Work out the finished part from the listing and answer in its coordinate system (mm). A direction names the side the tool comes from. Give positions to 0.01 mm unless a question says otherwise; leave off trailing zeros. Loops run counter-clockwise (first coordinate to the right, second up) from the corner with the lowest first, then second, coordinate; pieces in that order, holes last. Notation, with made-up numbers: (-25.5, -26) - (-11.5, -26) arc R24 cw to (-11.5, 10) - close; hole circle Ø5 at (52.25, 71.25). An arc over 180 degrees is marked (long way). Use CSV: the item, a comma, the result in double quotes.
from build123d import *

# Parameters (mm, degrees)
BOSS_EXTRU_1_DEPTH = 6.9
TROU_TARAUD_M81_D  = 6.8


with BuildPart() as part:
    # Esquisse1 → Boss.-Extru.1 (new body)
    with BuildSketch(Plane.XY):
        Polygon((-5.9, -3.406366588), (0, -6.812733176), (5.9, -3.406366588), (5.9, 3.406366588), (0, 6.812733176), (-5.9, 3.406366588), align=None)
    extrude(amount=BOSS_EXTRU_1_DEPTH)

    # Esquisse2 → Révolution1 (revolve)
    with BuildSketch(Plane(origin=(0, 0, 0), x_dir=(0, 0, -1), z_dir=(1, 0, 0)), mode=Mode.PRIVATE) as r_volution1_sk:
        Polygon((-1, 8.4), (-2.5, 5.801923789), (-2.5, 0), (0, 0), (0, 8.4), align=None)
    revolve(r_volution1_sk.sketch.rotate(Axis((0, 0, 0), (0, 0, 1)), 90), axis=Axis((0, 0, 0), (0, 0, 1)))

    # Esquisse3 → Enlèvement de matière-Révolution1 (revolve, cut)
    with BuildSketch(Plane(origin=(0, 0, 0), x_dir=(0, 0, -1), z_dir=(1, 0, 0))):
        Polygon((-6.9, 6.812733176), (-6.9, 5.946707773), (-6.4, 6.812733176), align=None)
    revolve(axis=Axis((0, 0, 0), (0, 0, 1)), mode=Mode.SUBTRACT)

    # Trou taraudé M81 (through all)
    with Locations(Plane.XY.offset(6.9)):
        with Locations((0, 0)):
            Hole(TROU_TARAUD_M81_D / 2)


solid = part.part
Item 1: The mould has two halves that part along Y. Classify faces 6 (the flat face through (-2.991, -5.086, 4.373)), 7 (the cylindrical face through (0.74, -3.32, 3.4)), 8 (the flat face through (-5.9, 0, 4)), 9 (the conical face through (5.381, 3.067, 6.758)): pulls with the +Y half, pulls with the -Y half, needs draft (parallel to the pull), parting line crosses it, or undercut.
Determined:
face 6,"pulls with the -Y half"
face 7,"undercut"
face 8,"needs draft"
face 9,"pulls with the +Y half"
Item 2: Given P1, Ø4, axis at y = -1, z = 4.5, coming from the -X side; P2, Ø1, axis at y = -1, z = 4, coming from the +X side; P3, Ø4, axis at y = -2, z = 3.5, coming from the -X side; P4, Ø8, axis at x = -1, y = -2, coming from the -Z side, each flat-ended and moving along its own axis, determine where each tip first touches the part or whether it passes through.
Determined:
P1,"stops at x = -5.9"
P2,"stops at x = 5.9"
P3,"stops at x = -7.3"
P4,"stops at z = 0"
Item 3: Find the intervals of material crossed by line 1 (X direction, y = -0.5, z = 1.75); line 2 (Z direction, x = 3.75, y = 6); line 3 (Y direction, x = 1.75, z = 2.5), in increasing order.
Determined:
line 1,"x = -7.08 to -3.36, 3.36 to 7.08"
line 2,"z = 0 to 1.76"
line 3,"y = -5.8 to -2.92, 2.92 to 5.8"
Item 4: For faces 1 (the flat face through (4, 0, 0)), 2 (the flat face through (-2.909, 5.133, 4.373)), 3 (the flat face through (2.991, 5.086, 4.373)), 4 (the cylindrical face through (-8.012, -2.523, 0.507)), 5 (the flat face through (2.909, -5.133, 4.373)), determine the directions among +Z, -Z, +X, -X, +Y, -Y from which every point of the face is accessible in a straight line to the end or side of a thin tool.
Determined:
face 1,"-Z, +X, -X, +Y, -Y"
face 2,"+Z, -X, +Y"
face 3,"+Z, +X, +Y"
face 4,"+Z, -Z"
face 5,"+Z, +X, -Y"
Item 5: A cutting plane is placed at A-A on y = 0. Determine the outline of the cut face in (x, z).
Determined:
outline,"(-8.4, 0) - (-3.4, 0) - (-3.4, 6.9) - (-5.9, 6.9) - (-5.9, 2.44) - (-8.4, 1) - close; (3.4, 0) - (8.4, 0) - (8.4, 1) - (5.9, 2.44) - (5.9, 6.9) - (3.4, 6.9) - close"
Item 6: A cutting plane is placed at C-C on z = 1.25. Determine the outline of the cut face in (x, y), and give its area (3 significant figures).
Determined:
outline,"circle Ø15.93 at (0, 0); hole circle Ø6.8 at (0, 0)"
area,"163 mm²"
Item 7: A cutting plane is placed at B-B on z = 2.75. Determine the outline of the cut face in (x, y).
Determined:
outline,"(-5.9, -3.41) - (0, -6.81) - (5.9, -3.41) - (5.9, 3.41) - (0, 6.81) - (-5.9, 3.41) - close; hole circle Ø6.8 at (0, 0)"
